Input: part model. Units: mm. Frame: model coordinates. A direction names the side the tool comes from. Round coordinates to 2 decimals unless told otherwise and drop trailing zeros. Order: outer loops, then holes, each group sorted by start corner. A loop starts at its lowest first (then second) coordinate and runs counter-clockwise, first axis right, second up.
Item 1: Cut plane C-C on y = -10. Output: boundary loops of the cut face in (x, z) (3 decimals).
Item 2: Cut plane B-B on x = -1. Output: boundary loops of the cut face in (y, z) (3 decimals).
Item 3: Mould query, pull axis X, two halves, no side actions, for faces 3 (the flat face through (-15.875, 0, 8)), 4 (the flat face through (12.7, 0, 9)), 5 (the flat face through (0, -15.875, 8)). Classes: released by +X, released by -X, zero draft, split by the parting line, or undercut.
Item 4: Cut plane A-A on z = 14. Output: boundary loops of the cut face in (x, y) (3 decimals), then the cut area to 3 significant figures.
Item 5: Reachability of faces 1 (the flat face through (15.875, 0, 8)), 2 (the flat face through (1, -12.7, 9)) from +Z, -Z, +X, -X, +Y, -Y: full face, straight path, thin tool, end or side. Return the list, or none.
Item 6: Line query: L1, parallel to X at y = -10, z = 7 (3 decimals); L2, parallel to X at y = 11.5, z = 6.25 (3 decimals); L3, parallel to Y at x = -5, z = 4.25 (3 decimals). Output: solid intervals per line, ascending.
```python
from build123d import *

# Parameters (mm, degrees)
F0_W     = 31.75
F0_H     = 31.75
F1_DEPTH = 3.175
F2_W     = 31.75
F2_H     = 31.75
F3_DEPTH = 12.7


# Not quite as in the source:
# - a length typed as a fraction of an inch, garbled in the dataset ("3 / 203.2 mm" for 3/8 in), is restored


with BuildPart() as f1:
    # F0 (on Top) → F1 (new body)
    with BuildSketch(Plane.XY):
        Rectangle(F0_W, F0_H)
    extrude(amount=F1_DEPTH)

    # F2 (on face) → F3 (join)
    with BuildSketch(Plane.XY.offset(3.175)):
        Rectangle(F2_W, F2_H)
        Polygon((12.7, 11.8309138343), (12.7, -12.7), (-11.8309138343, -12.7), (-12.7, -12.7), (-12.7, -11.8309138343), (-12.7, 12.7), (11.8309138343, 12.7), (12.7, 12.7), align=None, mode=Mode.SUBTRACT)
        Polygon((-12.7, -11.8309138343), (-12.7, -12.7), (12.7, 12.7), (11.8309138343, 12.7), align=None)
        Polygon((-12.7, -12.7), (-11.8309138343, -12.7), (12.7, 11.8309138343), (12.7, 12.7), align=None)
    extrude(amount=F3_DEPTH)


solid = f1.part
```
From the geometry:
1. outline: (-15.875, 0) - (15.875, 0) - (15.875, 15.875) - (12.7, 15.875) - (12.7, 3.175) - (-9.131, 3.175) - (-9.131, 15.875) - (-10.869, 15.875) - (-10.869, 3.175) - (-12.7, 3.175) - (-12.7, 15.875) - (-15.875, 15.875) - close
2. outline: (-15.875, 0) - (15.875, 0) - (15.875, 15.875) - (12.7, 15.875) - (12.7, 3.175) - (-0.131, 3.175) - (-0.131, 15.875) - (-1.869, 15.875) - (-1.869, 3.175) - (-12.7, 3.175) - (-12.7, 15.875) - (-15.875, 15.875) - close
3. face 3: released by -X
3. face 4: undercut
3. face 5: zero draft
4. outline: (-15.875, -15.875) - (15.875, -15.875) - (15.875, 15.875) - (-15.875, 15.875) - close; hole (-12.7, -11.831) - (11.831, 12.7) - (-12.7, 12.7) - close; hole (-11.831, -12.7) - (12.7, -12.7) - (12.7, 11.831) - close
4. area: 406 mm2
5. face 1: +Z, -Z, +X, +Y, -Y
5. face 2: +Z
6. L1: x = -15.875 to -12.7, -10.869 to -9.131, 12.7 to 15.875
6. L2: x = -15.875 to -12.7, 10.631 to 12.369, 12.7 to 15.875
6. L3: y = -15.875 to -12.7, -5.869 to -4.131, 12.7 to 15.875
